from build123d import *

# Parameters (mm, degrees)
SKETCH1_R                                       = 37.5
BOSS_EXTRUDE1_DEPTH                             = 6
SKETCH2_R                                       = 31.7
CUT_EXTRUDE1_DEPTH                              = 6
SKETCH3_W                                       = 85
SKETCH3_H                                       = 85
BOSS_EXTRUDE2_DEPTH                             = 25.4
FILLET2_R                                       = 4
SKETCH4_W                                       = 65
SKETCH4_H                                       = 65
CUT_EXTRUDE2_DEPTH                              = 16.51
CSK_FOR_M6_FLAT_HEAD_MACHINE_SCREW1_D           = 6.6
CSK_FOR_M6_FLAT_HEAD_MACHINE_SCREW1_CSINK_D     = 12.6
CSK_FOR_M6_FLAT_HEAD_MACHINE_SCREW1_CSINK_ANGLE = 90
SKETCH8_W                                       = 85
SKETCH8_H                                       = 85
CUT_EXTRUDE3_DEPTH                              = 16.51
SKETCH9_W                                       = 116
SKETCH9_H                                       = 87
SKETCH9_W_2                                     = 85
SKETCH9_H_2                                     = 85
BOSS_EXTRUDE3_DEPTH                             = 8.89
CUT_EXTRUDE4_DEPTH                              = 8.89
SKETCH11_W                                      = 26
SKETCH11_H                                      = 32.35
CUT_EXTRUDE5_DEPTH                              = 3
CUT_EXTRUDE6_DEPTH                              = 8.89
SKETCH14_R                                      = 1
CUT_EXTRUDE7_DEPTH                              = 8.89
FILLET3_R                                       = 3


with BuildPart() as part:
    # Sketch1 → Boss-Extrude1 (new body)
    with BuildSketch(Plane.XY):
        Circle(SKETCH1_R)
    extrude(amount=-BOSS_EXTRUDE1_DEPTH)

    # Sketch2 → Cut-Extrude1 (cut)
    with BuildSketch(Plane(origin=(0, 0, -6), x_dir=(-1, 0, 0), z_dir=(0, 0, -1))):
        Circle(SKETCH2_R)
    extrude(amount=-CUT_EXTRUDE1_DEPTH, mode=Mode.SUBTRACT)

    # Sketch3 → Boss-Extrude2 (add)
    with BuildSketch(Plane.XY):
        Rectangle(SKETCH3_W, SKETCH3_H)
    extrude(amount=BOSS_EXTRUDE2_DEPTH)

    # Fillet2
    fillet2_edges = [part.edges().sort_by_distance(p)[0] for p in [
        (-37.5, 0, 0),
    ]]
    fillet(fillet2_edges, radius=FILLET2_R)

    # Sketch4 → Cut-Extrude2 (cut)
    with BuildSketch(Plane.XY.offset(25.4)):
        Rectangle(SKETCH4_W, SKETCH4_H)
    extrude(amount=-CUT_EXTRUDE2_DEPTH, mode=Mode.SUBTRACT)

    # CSK for M6 Flat Head Machine Screw1 (through all)
    with Locations(Plane.XY.offset(8.89)):
        with Locations((-17.67766953, 17.67766953), (-17.67766953, -17.67766953), (17.67766953, -17.67766953), (17.67766953, 17.67766953)):
            CounterSinkHole(CSK_FOR_M6_FLAT_HEAD_MACHINE_SCREW1_D / 2, CSK_FOR_M6_FLAT_HEAD_MACHINE_SCREW1_CSINK_D / 2, counter_sink_angle=CSK_FOR_M6_FLAT_HEAD_MACHINE_SCREW1_CSINK_ANGLE)

    # Sketch8 → Cut-Extrude3 (cut)
    with BuildSketch(Plane.XY.offset(25.4)):
        Rectangle(SKETCH8_W, SKETCH8_H)
    extrude(amount=-CUT_EXTRUDE3_DEPTH, mode=Mode.SUBTRACT)

    # Sketch9 → Boss-Extrude3 (add)
    with BuildSketch(Plane.XY.offset(8.89)):
        with Locations((-14.5, 0)):
            Rectangle(SKETCH9_W, SKETCH9_H)
        Rectangle(SKETCH9_W_2, SKETCH9_H_2, mode=Mode.SUBTRACT)
    extrude(amount=-BOSS_EXTRUDE3_DEPTH)

    # Sketch12 → Cut-Extrude4 (cut)
    with BuildSketch(Plane.XY.offset(8.89)):
        Polygon((-42.5, -43.5), (-72.5, -18.5), (-72.5, -43.5), align=None)
    extrude(amount=-CUT_EXTRUDE4_DEPTH, mode=Mode.SUBTRACT)

    # Sketch11 → Cut-Extrude5 (cut)
    with BuildSketch(Plane.XY.offset(8.89)):
        with Locations((-54.5, 22.325)):
            Rectangle(SKETCH11_W, SKETCH11_H)
    extrude(amount=-CUT_EXTRUDE5_DEPTH, mode=Mode.SUBTRACT)

    # Sketch13 → Cut-Extrude6 (cut)
    with BuildSketch(Plane.XY.offset(8.89)):
        with BuildLine():
            Line((-49.5, -5.85), (-59.5, -5.85))
            ThreePointArc((-59.5, -5.85), (-61.5, -3.85), (-59.5, -1.85))
            Line((-59.5, -1.85), (-49.5, -1.85))
            ThreePointArc((-49.5, -1.85), (-47.5, -3.85), (-49.5, -5.85))
        make_face()
    extrude(amount=-CUT_EXTRUDE6_DEPTH, mode=Mode.SUBTRACT)

    # Sketch14 → Cut-Extrude7 (cut)
    with BuildSketch(Plane.XY.offset(8.89)):
        with Locations((38.5, -38.5)):
            Circle(SKETCH14_R)
        with Locations((38.5, 38.5)):
            Circle(SKETCH14_R)
        with Locations((-24.5, 38.5)):
            Circle(SKETCH14_R)
        with Locations((-44.898080814, -28.46206612)):
            Circle(SKETCH14_R)
    extrude(amount=-CUT_EXTRUDE7_DEPTH, mode=Mode.SUBTRACT)

    # Fillet3
    fillet3_edges = [part.edges().sort_by_distance(p)[0] for p in [
        (43.5, 43.5, 4.445),
        (43.5, -43.5, 4.445),
        (-72.5, 43.5, 4.445),
        (-72.5, -18.5, 4.445),
        (-42.5, -43.5, 4.445),
    ]]
    fillet(fillet3_edges, radius=FILLET3_R)


solid = part.part
Can you work these out from the model? Positions are in its coordinate system, mm. A direction names the side the tool comes from. Coordinates: 2 decimals unless noted, no trailing zeros. Write each loop counter-clockwise with the first axis right and the second up, starting at its lowest first coordinate (ties: lowest second). Pieces come first, ordered by that corner, then holes.
Q1. If we mould it in two halves opening along X, with no side actions, what happens to faces 4 (the face through (-15.06, -19.69, 2.9)), 5 (the face through (42.6, 42.64, 4.38)), 6 (the face through (-71.64, 42.6, 4.38)), 7 (the face through (-4.88, 37.18, -4.99))? For each: +X half, -X half, draft (parallel to the pull), parting line (faces both ways), or undercut.
Results found:
face 4: undercut
face 5: +X half
face 6: -X half
face 7: parting line
Q2. For P1, Ø4.5, axis at x = -57, z = 3, coming from the -Y side; P2, Ø0.9, axis at x = -59, z = 8, coming from the -Y side (3 decimals); P3, Ø1, axis at y = -25, z = -2.5, coming from the +X side; P4, Ø1.2, axis at x = -24.5, y = 38.5, coming from the +Z side, each with a flat end and sliding along its axis, tell me the tip position at first contact or that it passes through.
Results found:
P1: stops at y = -33.29
P2: stops at y = -30.125
P3: stops at x = 28.87
P4: passes through
Q3. Imagine slicing it at B-B, the plane x = 0. List the corners of the cut face in (y, z) for me.
Results found:
outline: (-43.5, 0) - (-41.5, 0) arc R4 cw to (-37.5, -4) - (-37.5, -6) - (-31.7, -6) - (-31.7, 0) - (31.7, 0) - (31.7, -6) - (37.5, -6) - (37.5, -4) arc R4 cw to (41.5, 0) - (43.5, 0) - (43.5, 8.89) - (-43.5, 8.89) - close
Q4. Imagine slicing it at A-A, the plane x = -51.5. List the corners of the cut face in (y, z) for me, plus the area to 3 significant figures.
Results found:
outline: (-36, 0) - (-5.85, 0) - (-5.85, 8.89) - (-36, 8.89) - close; (-1.85, 0) - (43.5, 0) - (43.5, 8.89) - (38.5, 8.89) - (38.5, 5.89) - (6.15, 5.89) - (6.15, 8.89) - (-1.85, 8.89) - close
area: 574 mm2
Q5. Please list where these lines run through material, in increasing order: L1, parallel to Y at x = 38.5, z = 6.75; L2, parallel to Y at x = -24.5, z = 3.5; L3, parallel to Y at x = -21, z = 8.
Results found:
L1: y = -43.5 to -39.5, -37.5 to 37.5, 39.5 to 43.5
L2: y = -43.5 to 37.5, 39.5 to 43.5
L3: y = -43.5 to -21.95, -13.41 to 13.41, 21.95 to 43.5
Q6. Imagine slicing it at C-C, the plane z = 4.5. Count the separate pieces of the cut face and the enclosed holes in it, plus the area to 3 significant figures.
Results found:
separate pieces: 1
enclosed holes: 9
area: 9,510 mm2
Q7. Which directions (+Z, -Z, +X, -X, +Y, -Y) give clear straight access to the entire face, cutting with the end or side of a thin tool? Please do faces 1 (the face through (-47.5, -3.8, 4.5)), 2 (the face through (-67.5, 22, 7)), 3 (the face through (-57.181, -31.266, 4.507)).
Results found:
face 1: +Z, -Z
face 2: +Z
face 3: +Z, -Z, -X, -Y
